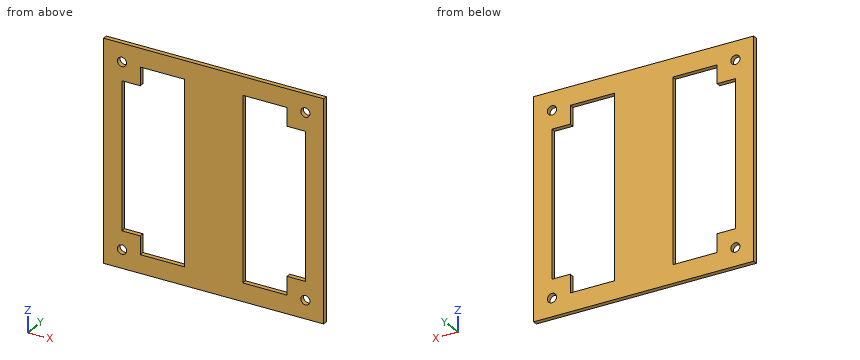
from build123d import *

# Parameters (mm, degrees)
SKETCH2_W           = 240
SKETCH2_H           = 240
BOSS_EXTRUDE1_DEPTH = 5
SKETCH3_W           = 63.5
SKETCH3_H           = 200
BOSS_EXTRUDE2_DEPTH = 5
SKETCH10_R          = 5
CUT_EXTRUDE1_DEPTH  = 10


with BuildPart() as part:
    # Sketch2 → Boss-Extrude1 (new body)
    with BuildSketch(Plane(origin=(0, 0, 0), x_dir=(1, 0, 0), z_dir=(0, 1, 0))):
        with Locations((0, 120)):
            Rectangle(SKETCH2_W, SKETCH2_H)
        Polygon((-100, 200), (-100, 40), (-80, 40), (-80, 20), (80, 20), (80, 40), (100, 40), (100, 200), (80, 200), (80, 220), (-80, 220), (-80, 200), align=None, mode=Mode.SUBTRACT)
    extrude(amount=-BOSS_EXTRUDE1_DEPTH)

    # Sketch3 → Boss-Extrude2 (add)
    with BuildSketch(Plane(origin=(0, 0, 0), x_dir=(1, 0, 0), z_dir=(0, 1, 0))):
        with Locations((0, 120)):
            Rectangle(SKETCH3_W, SKETCH3_H)
    extrude(amount=-BOSS_EXTRUDE2_DEPTH)

    # Sketch10 → Cut-Extrude1 (cut)
    with BuildSketch(Plane(origin=(0, 0, 0), x_dir=(1, 0, 0), z_dir=(0, 1, 0))):
        with Locations(Location((-100, 20, 0), (0, 0, 270))):
            Circle(SKETCH10_R)
        with Locations(Location((100, 20, 0), (0, 0, 270))):
            Circle(SKETCH10_R)
        with Locations(Location((-100, 220, 0), (0, 0, 270))):
            Circle(SKETCH10_R)
        with Locations(Location((100, 220, 0), (0, 0, 270))):
            Circle(SKETCH10_R)
    extrude(amount=-CUT_EXTRUDE1_DEPTH, mode=Mode.SUBTRACT)


solid = part.part
The model under review builds one solid part; all positions refer to its coordinate system, in mm. Round coordinates to 2 decimals unless told otherwise and drop trailing zeros. Order: outer loops, then holes, each group sorted by start corner. A loop starts at its lowest first (then second) coordinate and runs counter-clockwise, first axis right, second up. Notation, with made-up numbers: (68.5, 62) -> (88.5, 62) arc R20 cw to (88.5, 82) -> close; hole circle Ø5 at (-27, 9.25). An arc over 180 degrees is marked (long way). Write item = value, one per line. Start each with the question number.
Item 1: Clearance check with a flat-ended pin moving along its axis: pin 1 Ø1.5 at (x, y) = (14, -1) entering from +Z. State where the tip first meets the part, or that it passes through.
Item 2: Consider section A-A on y = -4. Write out the cut boundary in (x, z).
Item 3: Consider section B-B on z = -182. Write out the cut boundary in (x, y).
Item 4: For line 1 along X through (y, z) = (-1.4, -27); line 2 along X through (y, z) = (-4.3, -168); line 3 along Z through (x, y) = (-39, -3.4), list the stretches that pass through material, from the lowest coordinate up.
Conclusion:
q1.pin_1 = 0
q2.outline = (-120, -240) -> (120, -240) -> (120, 0) -> (-120, 0) -> close; hole circle Ø10 at (-100, -220); hole circle Ø10 at (-100, -20); hole (-100, -200) -> (-80, -200) -> (-80, -220) -> (-31.75, -220) -> (-31.75, -20) -> (-80, -20) -> (-80, -40) -> (-100, -40) -> close; hole (31.75, -220) -> (80, -220) -> (80, -200) -> (100, -200) -> (100, -40) -> (80, -40) -> (80, -20) -> (31.75, -20) -> close; hole circle Ø10 at (100, -220); hole circle Ø10 at (100, -20)
q3.outline = (-120, -5) -> (-100, -5) -> (-100, 0) -> (-120, 0) -> close; (-31.75, -5) -> (31.75, -5) -> (31.75, 0) -> (-31.75, 0) -> close; (100, -5) -> (120, -5) -> (120, 0) -> (100, 0) -> close
q4.line_1 = -120 to -80, -31.75 to 31.75, 80 to 120
q4.line_2 = -120 to -100, -31.75 to 31.75, 100 to 120
q4.line_3 = -240 to -220, -20 to 0
